Work out the finished part from the listing and answer in its coordinate system (mm). Face numbers are marked on the shaded views. A direction names the side the tool comes from. Coordinates: 2 decimals unless noted, no trailing zeros. Order: outer loops, then holes, each group sorted by start corner. A loop starts at its lowest first (then second) coordinate and runs counter-clockwise, first axis right, second up. Notation, with made-up numbers: M -38.75,88 L -29.75,88 A8 cw -29.75,102 Z; hole C 32.5,20.5 d7. An arc over 180 degrees is marked long. Answer in a Markdown table with one row per item. Add a question column.
Item 1: The part is cut by section B-B (y = 23). Write down the section's boundary in (x, z), then the cut area to 3 significant figures.
Item 2: Consider line 1 (X direction, y = 28, z = 15); line 2 (Z direction, x = -2.75, y = 34); line 3 (Y direction, x = 9, z = -2). Determine where each line is inside the solid, lowest interval first. Write a range as from..to.
Item 3: The mould has two halves that part along X. Classify the marked faces 3, 4, 5 and 6: released by +X, released by -X, zero draft, split by the parting line, or undercut.
Item 4: The part is cut by section C-C (z = 4). Write down the section's boundary in (x, y), then the cut area to 3 significant figures.
Item 5: Flat-ended cylindrical pins translate along their axes: pin 1 Ø3.5 at (x, z) = (-6.5, 33) entering from -Y; pin 2 Ø2 at (y, z) = (39.5, -21) entering from -X; pin 3 Ø9 at (x, z) = (-0.5, 7) entering from +Y. Find the tip coordinate at first contact, or state that the pin passes through.
Item 6: The part is cut by section A-A (x = 8.75). Write down the section's boundary in (y, z), then the cut area to 3 significant figures.
Item 7: The part is cut by section D-D (z = 20). Write down the section's boundary in (x, y), then the cut area to 3 significant figures.
Item 8: Which of the six approach directions +Z, -Z, +X, -X, +Y, -Y give full straight-line access (tool end or side, diameter ignored) to the marked faces 1 and 2?
Autodesk Inventor part; units mm, degrees
ref_plane "YZ Plane" through (0, 0, 0) normal (1, 0, 0) x (0, 1, 0)
ref_plane "XZ Plane" through (0, 0, 0) normal (0, 1, 0) x (-1, 0, 0)
ref_plane "XY Plane" through (0, 0, 0) normal (0, 0, 1) x (1, 0, 0)
sketch "Sketch1" plane through (0, 0, 0) normal (0, 1, 0) x (-1, 0, 0)
  line L0 (12.0626, 25.212) -> (-7.9374, 25.212)
  line L1 (-7.9374, 25.212) -> (-7.9374, -14.788)
  line L2 (-7.9374, -14.788) -> (12.0626, -14.788)
  line L3 (12.0626, -14.788) -> (12.0626, 25.212)
  line L4 (12.0626, 25.212) -> (-7.9374, -14.788) construction
  line L5 (-7.9374, 25.212) -> (12.0626, -14.788) construction
  point P0 (0, 0)
  point P1 (2.0626, 5.212)
  dimension "d0" = 20
  dimension "d1" = 40
extrude "Extrusion1" add sketch "Sketch1" along normal blind 3
sketch "Sketch2" plane through (0, 3, 0) normal (0, 1, 0) x (1, 0, 0)
  line L0 (-15.0626, -28.212) -> (10.9374, -28.212)
  line L1 (10.9374, -28.212) -> (10.9374, 17.788)
  line L2 (10.9374, 17.788) -> (-15.0626, 17.788)
  line L3 (-15.0626, 17.788) -> (-15.0626, -28.212)
  line L4 (-15.0626, -28.212) -> (10.9374, 17.788) construction
  line L5 (10.9374, -28.212) -> (-15.0626, 17.788) construction
  line L6 (-12.0626, 14.788) -> (-12.0626, -25.212)
  line L7 (-12.0626, -25.212) -> (7.9374, -25.212)
  line L8 (7.9374, 14.788) -> (-12.0626, 14.788)
  line L9 (-12.0626, 14.788) -> (-12.0626, -25.212)
  line L10 (-12.0626, -25.212) -> (7.9374, -25.212)
  line L11 (7.9374, -25.212) -> (7.9374, 14.788)
  line L12 (7.9374, 14.788) -> (-12.0626, -25.212) construction
  line L13 (-12.0626, 14.788) -> (7.9374, -25.212) construction
  point P0 (0, 0)
  point P1 (-2.0626, -5.212)
  point P2 (7.9374, -25.212)
  dimension "d4" = 26
  dimension "d5" = 46
  dimension "d6" = 3
  dimension "d7" = 3
extrude "Extrusion2" add sketch "Sketch2" along normal blind 38 and the other way blind 3
fillet "Fillet1" radius 1 13 edges at (10.9374, 0, 5.212) (-2.0626, 0, -17.788) (10.9374, 20.5, -17.788) (-15.0626, 20.5, -17.788) (-15.0626, 0, 5.212) (10.9374, 20.5, 28.212) (-15.0626, 20.5, 28.212) (-12.0626, 22, -14.788) (-12.0626, 3, 5.212) (7.9374, 3, 5.212) (7.9374, 22, -14.788) (7.9374, 22, 25.212) (-12.0626, 22, 25.212)
sketch "Sketch8" plane through (10.9374, 1, 27.212) normal (1, 0, 0) x (0, 0, -1)
  line L0 (32, 7) -> (22, 7)
  line L1 (22, 7) -> (22, 13)
  line L2 (22, 13) -> (32, 13)
  line L3 (32, 13) -> (32, 7)
  line L4 (-1, -1) -> (44, -1)
  line L5 (45, 0) -> (45, 40)
  point P0 (27.212, -1)
  point P1 (27, 7)
  dimension "d25" = 10
  dimension "d26" = 6
  dimension "d27" = 8
  dimension "d28" = 13
extrude "Extrusion4" cut sketch "Sketch8" against normal blind 3
sketch "Sketch9" plane through (0, 0, 0) normal (0, -1, 0) x (1, 0, 0)
  circle A0 centre (-2.0626, -5.288) radius 6.5
  line L0 (-14.0626, -17.788) -> (9.9374, -17.788)
  line L1 (10.9374, -16.788) -> (10.9374, 27.212)
  point P0 (0, 0)
  dimension "d31" = 13
  dimension "d32" = 12.5
  dimension "d36" = 13
extrude "Extrusion5" cut sketch "Sketch9" against normal blind 3
sketch "Sketch11" plane through (-14.0626, 0, 28.212) normal (0, 0, 1) x (1, 0, 0)
  line L0 (19.4055, 36.5) -> (3.4055, 36.5)
  line L1 (3.4055, 36.5) -> (3.4055, 41)
  line L2 (3.4055, 41) -> (19.4055, 41)
  line L3 (19.4055, 41) -> (19.4055, 36.5)
  line L4 (0, 41) -> (24, 41)
  point P0 (14.0626, 0)
  point P1 (11.4055, 41)
  dimension "d37" = 16
  dimension "d38" = 4.5
  dimension "d39" = 0
extrude "Extrusion6" add sketch "Sketch11" along normal blind 7
chamfer "Chamfer1" distance 2 angle 45 2 edges at (-10.6572, 38.75, 35.212) (5.3428, 38.75, 35.212)
sketch "Sketch12" plane through (-10.6572, 36.5, 28.212) normal (0, -1, 0) x (1, 0, 0)
  point P0 (10.6572, -28.212)
sketch "Sketch13" plane through (-10.6572, 36.5, 28.212) normal (0, -1, 0) x (1, 0, 0)
  circle A0 centre (12, 4) radius 1.5
  circle A1 centre (4, 4) radius 1.5
  line L0 (16, 0) -> (16, 5)
  line L1 (2, 7) -> (14, 7)
  line L2 (0, 0) -> (0, 5)
  point P0 (10.6572, -28.212)
  dimension "d45" = 3
  dimension "d46" = 3
  dimension "d47" = 4
  dimension "d48" = 3
  dimension "d49" = 4
  dimension "d50" = 3
extrude "Extrusion7" cut sketch "Sketch13" against normal blind 7
ref_plane "Work Plane1" through (-14.0626, 0, 5.212) normal (0, 0, 1) x (1, 0, 0)
mirror "Mirror1" about plane through (-14.0626, 0, 5.212) normal (0, 0, 1) of "Extrusion6", "Extrusion7", "Chamfer1"
properties part number "servo_holder"
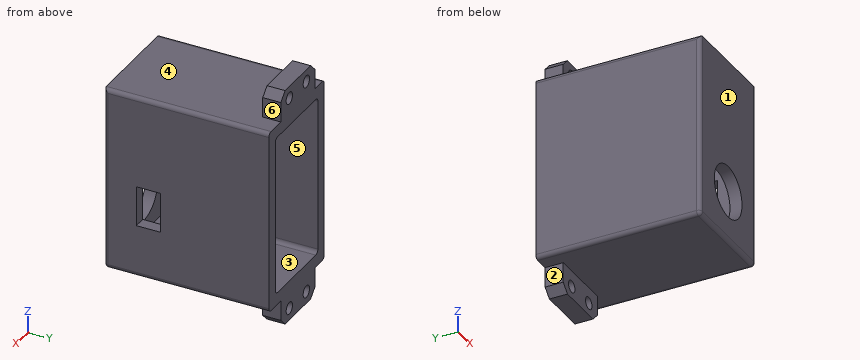
Reply:
| question | item | result |
|---|---|---|
| 1 | outline | M -15.06,-16.79 A1 ccw -14.06,-17.79 L 9.94,-17.79 A1 ccw 10.94,-16.79 L 10.94,27.21 A1 ccw 9.94,28.21 L -14.06,28.21 A1 ccw -15.06,27.21 Z; hole M -12.06,-13.79 A1 ccw -11.06,-14.79 L 6.94,-14.79 A1 ccw 7.94,-13.79 L 7.94,24.21 A1 ccw 6.94,25.21 L -11.06,25.21 A1 ccw -12.06,24.21 Z |
| 1 | area | 396 mm2 |
| 2 | line 1 | x = -15.06..-12.06, 7.94..10.94 |
| 2 | line 2 | z = -17.79..-14.79, 25.21..28.21 |
| 2 | line 3 | y = 0..8, 14..41 |
| 3 | face 3 | undercut |
| 3 | face 4 | zero draft |
| 3 | face 5 | undercut |
| 3 | face 6 | released by +X |
| 4 | outline | M -15.06,1 A1 ccw -14.06,0 L 9.94,0 A1 ccw 10.94,1 L 10.94,8 L 7.94,8 L 7.94,4 A1 cw 6.94,3 L -11.06,3 A1 cw -12.06,4 L -12.06,41 L -15.06,41 Z; M 7.94,14 L 10.94,14 L 10.94,41 L 7.94,41 Z |
| 4 | area | 288 mm2 |
| 5 | pin 1 | stops at y = 36.5 |
| 5 | pin 2 | stops at x = -10.66 |
| 5 | pin 3 | stops at y = 3 |
| 6 | outline | M 0,-16.79 A1 ccw 1,-17.79 L 41,-17.79 L 41,28.21 L 0,28.21 Z; hole M 8,-4.79 L 14,-4.79 L 14,5.21 L 8,5.21 Z |
| 6 | area | 1,830 mm2 |
| 7 | outline | M -15.06,1 A1 ccw -14.06,0 L 9.94,0 A1 ccw 10.94,1 L 10.94,41 L 7.94,41 L 7.94,4 A1 cw 6.94,3 L -11.06,3 A1 cw -12.06,4 L -12.06,41 L -15.06,41 Z |
| 7 | area | 306 mm2 |
| 8 | face 1 | +Z, -Z, +X, -X, -Y |
| 8 | face 2 | -Z, -X, +Y, -Y |
